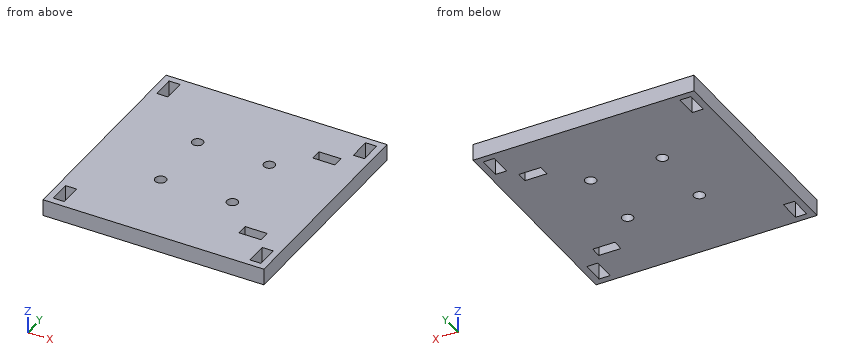
from build123d import *

# Parameters (mm, degrees)
SKETCH1_W           = 40
SKETCH1_H           = 40
SKETCH1_R           = 1
BOSS_EXTRUDE1_DEPTH = 3
SKETCH2_W           = 2
SKETCH2_H           = 4
SKETCH2_W_2         = 4
SKETCH2_H_2         = 2
CUT_EXTRUDE1_DEPTH  = 29.442925307


with BuildPart() as part:
    # Sketch1 → Boss-Extrude1 (new body)
    with BuildSketch(Plane.XY):
        Rectangle(SKETCH1_W, SKETCH1_H)
        with Locations((6.5, -6)):
            Circle(SKETCH1_R, mode=Mode.SUBTRACT)
        with Locations(Location((-6.5, -6, 0), (0, 0, 180))):
            Circle(SKETCH1_R, mode=Mode.SUBTRACT)
        with Locations(Location((6.5, 6, 0), (0, 0, 180))):
            Circle(SKETCH1_R, mode=Mode.SUBTRACT)
        with Locations((-6.5, 6)):
            Circle(SKETCH1_R, mode=Mode.SUBTRACT)
    extrude(amount=BOSS_EXTRUDE1_DEPTH)

    # Sketch2 → Cut-Extrude1 (cut, through all)
    with BuildSketch(Plane.XY.offset(3)):
        with Locations((17.8, 16.8)):
            Rectangle(SKETCH2_W, SKETCH2_H)
        with Locations((-17.8, 16.8)):
            Rectangle(SKETCH2_W, SKETCH2_H)
        with Locations((13.6, 12)):
            Rectangle(SKETCH2_W_2, SKETCH2_H_2)
        with Locations((17.8, -16.8)):
            Rectangle(SKETCH2_W, SKETCH2_H)
        with Locations((-17.8, -16.8)):
            Rectangle(SKETCH2_W, SKETCH2_H)
        with Locations((13.6, -12)):
            Rectangle(SKETCH2_W_2, SKETCH2_H_2)
    extrude(amount=-CUT_EXTRUDE1_DEPTH, mode=Mode.SUBTRACT)


solid = part.part
The listing builds one solid part. Answer for the finished solid, in the listing's coordinates (mm). Round coordinates to 2 decimals unless told otherwise and drop trailing zeros. Loops run counter-clockwise (first coordinate to the right, second up) from the corner with the lowest first, then second, coordinate; pieces in that order, holes last. Notation, with made-up numbers: M 75,-22.5 L 87,-22.5 A30 cw 87,9.5 Z; hole C -3.75,79 d9. An arc over 180 degrees is marked long. Return JSON: item names as keys, results as strings.
Q1. Find section B-B, the plane x = -6.5. Determine the outline of the cut face in (y, z).
Results list:
{"outline": "M -20,0 L -7,0 L -7,3 L -20,3 Z; M -5,0 L 5,0 L 5,3 L -5,3 Z; M 7,0 L 20,0 L 20,3 L 7,3 Z"}
Q2. Find section C-C, the plane z = 1.9. State how many separate pieces and enclosed holes the cut face has, plus the area to 3 significant figures.
Results list:
{"separate pieces": "1", "enclosed holes": "10", "area": "1,540 mm2"}
Q3. This flat-tipped pin is pushed along its axis until it touches: pin 1 Ø1.8 at (x, y) = (6.5, -6) entering from -Z. Where does it stop, or does it pass through?
Results list:
{"pin 1": "passes through"}
Q4. Find section A-A, the plane y = 6. Determine the outline of the cut face in (x, z), plus the area to 3 significant figures.
Results list:
{"outline": "M -20,0 L -7.5,0 L -7.5,3 L -20,3 Z; M -5.5,0 L 5.5,0 L 5.5,3 L -5.5,3 Z; M 7.5,0 L 20,0 L 20,3 L 7.5,3 Z", "area": "108 mm2"}
Q5. Find the intervals of material crossed by line 1 along Y through (x, z) = (6.5, 1.3); line 2 along Y through (x, z) = (17.5, 0.8); line 3 along X through (y, z) = (-6.5, 1.05), in increasing order. Write a range as from..to.
Results list:
{"line 1": "y = -20..-7, -5..5, 7..20", "line 2": "y = -20..-18.8, -14.8..14.8, 18.8..20", "line 3": "x = -20..-7.37, -5.63..5.63, 7.37..20"}
